The drawing under review shows one solid part. Ordinate dimensions are in mm from its lowest x, y, z. A direction names the side the tool comes from. Coordinates: 2 decimals unless noted, no trailing zeros. Write each loop counter-clockwise with the first axis right and the second up, starting at its lowest first coordinate (ties: lowest second). Pieces come first, ordered by that corner, then holes.
Q1. Machinability: for the marked faces 1 and 2, which of the approach directions +Z, -Z, +X, -X, +Y, -Y give a long, thin tool a straight path to every point of the face, cutting with its end or side? Answer none if there is none.
Q2. Add section A-A, the plane x = 3.6. Give the boundary of the cut face in (y, z).
Q3. Clearance check with a flat-ended pin moving along its axis: pin 1 Ø1 at (y, z) = (6.5, 2) entering from +X. State where the tip first meets the part, or that it passes through.
Q4. Add section C-C, the plane z = 1.45. Give the boundary of the cut face in (x, y).
Q5. The part is to be moulded in two halves that separate along Y. For the marked faces 3, 4 and 5, say which applies: +Y half, -Y half, draft (parallel to the pull), parting line (faces both ways), or undercut.
Q6. To check wall thickness, follow probe 1 along Y at (x, z) = (3.6, 1.1); probe 2 along X at (y, z) = (3.75, 1.2); probe 3 along X at (y, z) = (4.5, 1.25). State the ranges of each line that lie inside material, in increasing order.
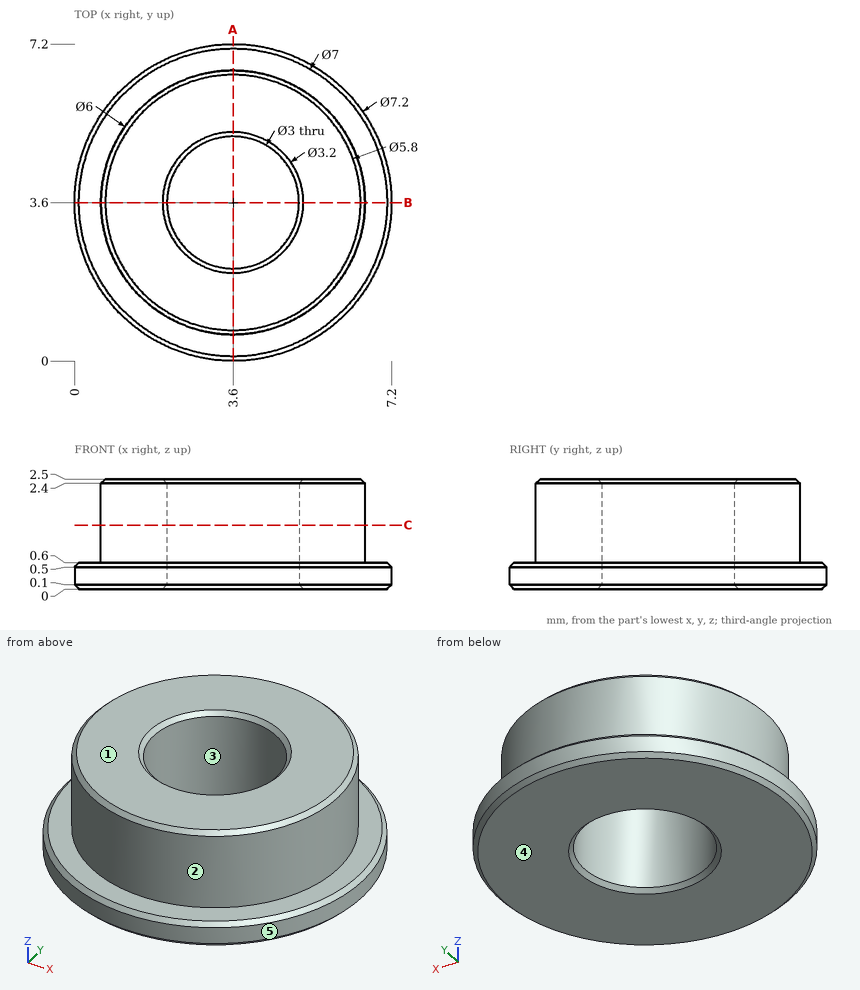
Here are the results:
1. face 1: +Z, +X, -X, +Y, -Y
1. face 2: +Z
2. outline: (0, 0.1) - (0.1, 0) - (2, 0) - (2.1, 0.1) - (2.1, 2.4) - (2, 2.5) - (0.7, 2.5) - (0.6, 2.4) - (0.6, 0.6) - (0.1, 0.6) - (0, 0.5) - close; (5.1, 0.1) - (5.2, 0) - (7.1, 0) - (7.2, 0.1) - (7.2, 0.5) - (7.1, 0.6) - (6.6, 0.6) - (6.6, 2.4) - (6.5, 2.5) - (5.2, 2.5) - (5.1, 2.4) - close
3. pin 1: stops at x = 5.4
4. outline: circle Ø6 at (3.6, 3.6); hole circle Ø3 at (3.6, 3.6)
5. face 3: undercut
5. face 4: draft
5. face 5: parting line
6. probe 1: y = 0.6 to 2.1, 5.1 to 6.6
6. probe 2: x = 0.6 to 2.11, 5.09 to 6.6
6. probe 3: x = 0.74 to 2.4, 4.8 to 6.46
